Autodesk Inventor part; units mm, degrees
ref_plane "YZ Plane" through (0, 0, 0) normal (1, 0, 0) x (0, 1, 0)
ref_plane "XZ Plane" through (0, 0, 0) normal (0, 1, 0) x (-1, 0, 0)
ref_plane "XY Plane" through (0, 0, 0) normal (0, 0, 1) x (1, 0, 0)
sketch "Sketch1" plane through (0, 0, 0) normal (0, 1, 0) x (-1, 0, 0)
  line L0 (0, 0) -> (150, 0)
  line L1 (150, 0) -> (150, -170)
  line L2 (150, -170) -> (0, -170)
  line L3 (0, -170) -> (0, 0)
  dimension "d0" = 150
  dimension "d1" = 170
extrude "Extrusion1" add sketch "Sketch1" along normal blind 5
sketch "Sketch2" plane through (0, 5, 0) normal (0, 1, 0) x (1, 0, 0)
  line L0 (-150, 170) -> (-150, 0)
  line L1 (-150, 0) -> (0, 0)
  line L2 (0, 0) -> (0, 170)
  line L3 (0, 170) -> (-150, 170)
  circle A0 centre (-117, 137) radius 2.75
  circle A1 centre (-140.5, 160.5) radius 1.75
  circle A2 centre (-140.5, 113.5) radius 1.75
  circle A3 centre (-93.5, 160.5) radius 1.75
  circle A4 centre (-93.5, 113.5) radius 1.75
  circle A5 centre (-45, 137) radius 2.75
  circle A6 centre (-10, 157) radius 2.75
  circle A7 centre (-115, 47.5) radius 2.75
  circle A8 centre (-95, 47.5) radius 2.75
  circle A9 centre (-135, 47.5) radius 2.75
  circle A10 centre (-45, 97) radius 2.75
  circle A11 centre (-45, 57) radius 2.75
  circle A12 centre (-45, 17) radius 2.75
  circle A13 centre (-10, 117) radius 2.75
  circle A14 centre (-10, 77) radius 2.75
  circle A15 centre (-10, 37) radius 2.75
  dimension "d5" = 5.5
  dimension "d8" = 3.5
  dimension "d9" = 9.5
  dimension "d10" = 9.5
  dimension "d13" = 47
  dimension "d16" = 47
  dimension "d23" = 5.5
  dimension "d24" = 5.5
  dimension "d25" = 33
  dimension "d26" = 13
  dimension "d28" = 170
  dimension "d36" = 10
  dimension "d40" = 45
  dimension "d43" = 5.5
  dimension "d44" = 5.5
  dimension "d48" = 20
  dimension "d49" = 35
  dimension "d50" = 5.5
  dimension "d51" = 20
  dimension "d53" = 23.5
  dimension "d54" = 23.5
  dimension "d55" = 33
  dimension "d58" = 40
  dimension "d65" = 40
extrude "Extrusion3" cut sketch "Sketch2" against normal blind 10 contours A0 | A1 | A2 | A3 | A4 | A5 | A6 | A7 | A8 | A9 | A10 | A11 | A12 | A13 | A14 | A15
equation "\"d16\" = d13"
equation "\"d36\" = d34"
equation "\"d40\" = d37"
equation "\"d53\" = 0.5 * d13"
equation "\"d54\" = d53"
properties part number "HeadPlate" material "Steel, Carbon"
Check sheet for the modelled part. Datum: model origin and axes. Units: mm. Give positions to 0.01 mm unless a question says otherwise; leave off trailing zeros. Loops run counter-clockwise (first coordinate to the right, second up) from the corner with the lowest first, then second, coordinate; pieces in that order, holes last. Notation, with made-up numbers: M 61.25,31.5 L 100.25,31.5 A20 cw 100.25,35.5 Z; hole C -30.5,-22.75 d9. An arc over 180 degrees is marked long. Return JSON: item names as keys, results as strings. Group by question number.
1. Cross-section at B-B on z = -77. Record the boundary of the cut face in (x, y), plus the area to 4 significant figures.
2. Cross-section at C-C on x = -10. Record the boundary of the cut face in (y, z), plus the area to 3 significant figures.
3. Mould release check, pull along X, two halves, no side actions. Record for faces 1 (the flat face through (-150, 2, -84)), 2 (the flat face through (-74, 0, -84)), 3 (the cylindrical face through (-10.358, 2.535, -39.727)), 4 (the cylindrical face through (-138.831, 2.535, -161.026)): released by +X, released by -X, zero draft, split by the parting line, or undercut.
4. Thickness scan on L1, parallel to Z at x = -10, y = 1.9; L2, parallel to Z at x = -45, y = 3.1; L3, parallel to X at y = 1.8, z = -137. Record the ranges inside material, lowest first.
5. Cross-section at A-A on x = -135. Record the boundary of the cut face in (y, z), plus the area to 4 significant figures.
6. Go/stop test with a flat-tipped pin: pin 1 (4.5 mm diameter, centred on x = -45, z = -137, fed in from +Y). Record where the tip stops, or that it passes through.
Return value:
{
 "1": {"outline": "M -150,0 L -12.75,0 L -12.75,5 L -150,5 Z; M -7.25,0 L 0,0 L 0,5 L -7.25,5 Z", "area": "722.5 mm^2"},
 "2": {"outline": "M 0,-170 L 5,-170 L 5,-159.75 L 0,-159.75 Z; M 0,-154.25 L 5,-154.25 L 5,-119.75 L 0,-119.75 Z; M 0,-114.25 L 5,-114.25 L 5,-79.75 L 0,-79.75 Z; M 0,-74.25 L 5,-74.25 L 5,-39.75 L 0,-39.75 Z; M 0,-34.25 L 5,-34.25 L 5,0 L 0,0 Z", "area": "740 mm^2"},
 "3": {"face 1": "released by -X", "face 2": "zero draft", "face 3": "undercut", "face 4": "undercut"},
 "4": {"L1": "-170 to -159.75, -154.25 to -119.75, -114.25 to -79.75, -74.25 to -39.75, -34.25 to 0", "L2": "-170 to -139.75, -134.25 to -99.75, -94.25 to -59.75, -54.25 to -19.75, -14.25 to 0", "L3": "-150 to -119.75, -114.25 to -47.75, -42.25 to 0"},
 "5": {"outline": "M 0,-170 L 5,-170 L 5,-50.25 L 0,-50.25 Z; M 0,-44.75 L 5,-44.75 L 5,0 L 0,0 Z", "area": "822.5 mm^2"},
 "6": {"pin 1": "through"}
}
